Autodesk Inventor part; units mm, degrees
ref_plane "YZ Plane" through (0, 0, 0) normal (1, 0, 0) x (0, 1, 0)
ref_plane "XZ Plane" through (0, 0, 0) normal (0, 1, 0) x (-1, 0, 0)
ref_plane "XY Plane" through (0, 0, 0) normal (0, 0, 1) x (1, 0, 0)
sketch "Sketch1" plane through (0, 0, 0) normal (0, 1, 0) x (-1, 0, 0)
  line L0 (30, 0) -> (0, 0)
  line L1 (3, 0) -> (3, 43.3)
  line L2 (3, 43.3) -> (21, 43.3)
  line L3 (21, 43.3) -> (21, 0)
  line L4 (15, -19.2684) -> (15, 39.5149) construction
  line L5 (8, 5) -> (16, 5)
  line L6 (16, 5) -> (16, 0)
  line L7 (8, 0) -> (8, 5)
  line L8 (7, 55) -> (7, 57.75)
  line L9 (7, 57.75) -> (17, 57.75)
  line L10 (17, 57.75) -> (17, 55)
  line L11 (0, 55) -> (7, 55)
  line L12 (17, 55) -> (30, 55)
  line L13 (0, 0) -> (0, 55)
  line L14 (30, 55) -> (30, 0)
  line L15 (7, 0) -> (7, -2.75)
  line L16 (7, -2.75) -> (17, -2.75)
  line L17 (17, -2.75) -> (17, 0)
  line L18 (0, 35) -> (-2.75, 35)
  line L19 (-2.75, 35) -> (-2.75, 20)
  line L20 (-2.75, 20) -> (0, 20)
  line L21 (25, 14.75) -> (25, 23.25)
  line L22 (25, 23.25) -> (24, 23.25)
  line L23 (24, 23.25) -> (24, 14.75)
  line L24 (24, 14.75) -> (25, 14.75)
  line L25 (24, 31.75) -> (25, 31.75)
  line L26 (25, 31.75) -> (25, 40.25)
  line L27 (25, 40.25) -> (24, 40.25)
  line L28 (24, 40.25) -> (24, 31.75)
  line L29 (12, 13) -> (12, 28.6373) construction
  point P0 (0, 0)
  point P1 (0, 0)
  point P2 (0, 0)
  point P3 (0, 0)
  point P4 (25.5, 44.5)
  point P5 (25.5, 27.5)
  point P6 (25.5, 10.5)
  dimension "d47" = 18
  dimension "d49" = 43.3
  dimension "d50" = 5
  dimension "d51" = 8
  dimension "d52" = 30
  dimension "d53" = 55
  dimension "d123" = 10
  dimension "d126" = 2.75
  dimension "d134" = 10
  dimension "d136" = 2.75
  dimension "d146" = 2.75
  dimension "d151" = 8.5
  dimension "d153" = 1
  dimension "d155" = 5
  dimension "d156" = 3
  dimension "d157" = 7
  dimension "d158" = 10.5
  dimension "d159" = 17
  dimension "d160" = 17
  dimension "d161" = 4.25
  dimension "d162" = 4.25
  dimension "d171" = 13
  dimension "d172" = 7
  dimension "d173" = 20
  dimension "d174" = 20
  dimension "d175" = 15
  dimension "d176" = 4.5
extrude "Extrusion1" add sketch "Sketch1" along normal blind 1.5
extrude "Extrusion2" add sketch "Sketch1" along normal blind 6 contours L0 L6 L5 L7 L1 L2 L3 | L0 L7 L5 L6
sketch "Sketch2" plane through (0, 0, 0) normal (0, 0, -1) x (-1, 0, 0)
  line L0 (8, 10) -> (16, 10)
  line L1 (16, 10) -> (16, 6)
  line L2 (16, 6) -> (8, 6)
  line L3 (8, 6) -> (8, 10)
  line L4 (0, 0) -> (7, 0)
  line L5 (16, 6) -> (16, 10)
  line L6 (12, 9) -> (12, -2.5232) construction
  line L7 (3, 1.5) -> (3, 6)
  line L8 (7, 1.5) -> (17, 1.5)
  point P0 (30, 0)
  point P1 (21.75, 6)
  point P2 (12, 1.5)
  dimension "d100" = 4
  dimension "d101" = 8
extrude "Extrusion7" add sketch "Sketch2" along normal blind 1.5
extrude "Extrusion9" cut sketch "Sketch1" along normal blind 10 contours L0 L7 L5 L6
extrude "Extrusion10" add sketch "Sketch1" along normal blind 10 contours L0 L7 L5 L6
hole "Hole1" at (-25.5, 0, 44.5) at (-25.5, 0, 27.5) at (-25.5, 0, 10.5) direction (0, 1, 0) diameter 1 end through all
properties part number "Motherboard_dummy" material "ABS Plastic"
Can you work these out from the model? Positions are in its coordinate system, mm. A direction names the side the tool comes from. Round coordinates to 2 decimals unless told otherwise and drop trailing zeros. Loops run counter-clockwise (first coordinate to the right, second up) from the corner with the lowest first, then second, coordinate; pieces in that order, holes last. Notation, with made-up numbers: M 75,55 L 124,55 A19 ccw 124,73 Z; hole C 34,1 d3. An arc over 180 degrees is marked long. Write item = value, one per line. Start each with the question number.
(1) Suppose I cut it at D-D on z = 25.5. Write out the boundary of the cut face in (x, y), plus the area to 3 significant figures.
(2) Suppose I cut it at B-B on y = 0.75. Write out the boundary of the cut face in (x, z), plus the area to 3 significant figures.
(3) Suppose I cut it at C-C on x = -9.5. Write out the boundary of the cut face in (y, z), plus the area to 3 significant figures.
(4) Which directions (+Z, -Z, +X, -X, +Y, -Y) give clear straight access to the entire face, cutting with the end or side of a thin tool? Please do faces 1 (the face through (-17, 1, -1)), 2 (the face through (-3, 4, 21)), 3 (the face through (-24, 1, 19)), 4 (the face through (0, 1, 10)), 5 (the face through (-3, 1, 55)).
(5) I need wall thicknesses on line 1 along Z through (x, y) = (-25.5, 1.1); line 2 along X through (y, z) = (1, 10.5); line 3 along X through (y, z) = (1, 37). Which ranges of each line are inside material? Lowest first, please.
(6) If we mould it in two halves opening along Y, with no side actions, what happens to faces 6 (the face through (-7, 1, -1)), 7 (the face through (-12, 10, 2)), 8 (the face through (-12, 1.5, -1))? For each: released by +Y, released by -Y, zero draft, split by the parting line, or undercut.
(7) I'm going to push flat-ended pins straight in: P1, Ø3, axis at x = -11, y = 8, coming from the +Z side; P2, Ø0.8, axis at y = 1, z = 55.5, coming from the -X side; P3, Ø1.6, axis at x = -26.5, y = 0.5, coming from the +Z side. Where does each tip first touch, or does it pass through?
(8) Suppose I cut it at A-A on z = 36. Write out the boundary of the cut face in (x, y).
Answer block:
q1.outline = M -30,0 L 2.75,0 L 2.75,1.5 L -3,1.5 L -3,6 L -21,6 L -21,1.5 L -30,1.5 Z
q1.area = 130 mm²
q2.outline = M -30,0 L -17,0 L -17,-2.75 L -7,-2.75 L -7,0 L 0,0 L 0,20 L 2.75,20 L 2.75,35 L 0,35 L 0,55 L -7,55 L -7,57.75 L -17,57.75 L -17,55 L -30,55 Z; hole C -25.5,10.5 d1; hole C -25.5,27.5 d1; hole C -25.5,44.5 d1; hole M -25,14.75 L -24,14.75 L -24,23.25 L -25,23.25 Z; hole M -25,31.75 L -24,31.75 L -24,40.25 L -25,40.25 Z
q2.area = 1,730 mm²
q3.outline = M 0,-2.75 L 1.5,-2.75 L 1.5,0 L 6,0 L 6,-1.5 L 10,-1.5 L 10,5 L 6,5 L 6,43.3 L 1.5,43.3 L 1.5,57.75 L 0,57.75 Z
q3.area = 312 mm²
q4.face_1 = -Z, -X, +Y, -Y
q4.face_2 = +Z, -Z, +X, +Y
q4.face_3 = +Y, -Y
q4.face_4 = -Z, +X, +Y, -Y
q4.face_5 = +Z, +X, +Y, -Y
q5.line_1 = 0 to 10, 11 to 27, 28 to 44, 45 to 55
q5.line_2 = -30 to -26, -25 to 0
q5.line_3 = -30 to -25, -24 to 0
q6.face_6 = zero draft
q6.face_7 = released by +Y
q6.face_8 = undercut
q7.P1 = 5
q7.P2 = -17
q7.P3 = 55
q8.outline = M -30,0 L -25,0 L -25,1.5 L -30,1.5 Z; M -24,0 L 0,0 L 0,1.5 L -3,1.5 L -3,6 L -21,6 L -21,1.5 L -24,1.5 Z
